Design review of the part shown in the three views and the two pictorial views. Dimensions are in mm from the part's minimum x, y and z. A direction names the side the tool comes from. Round coordinates to 2 decimals unless told otherwise and drop trailing zeros. Loops run counter-clockwise (first coordinate to the right, second up) from the corner with the lowest first, then second, coordinate; pieces in that order, holes last. Notation, with made-up numbers: (20.5, 74.5) -> (48.5, 74.5) arc R20 cw to (48.5, 81.5) -> close; hole circle Ø4 at (-35.5, -15). An arc over 180 degrees is marked (long way). Write each question's results on one line, items separated by ' | '. Start each with the question number.
Item 1: Clearance check with flat-ended pins moving along their axes: pin 1 Ø1.5 at (x, y) = (1.5, 18) entering from -Z; pin 2 Ø1.5 at (x, y) = (1, 18) entering from +Z; pin 3 Ø0.5 at (x, z) = (2, 0.5) entering from +Y. State where each tip first meets the part, or that it passes through.
Item 2: We need section A-A (z = 8). Give the boundary of the cut face in (x, y).
Item 3: Tool access review of the marked faces 1, 2, 3, 4 and 5: name each direction out of +Z, -Z, +X, -X, +Y, -Y from which nothing blocks a thin tool from reaching the whole face with its end or side.
Item 4: For L1, parallel to Y at x = 1.1, z = 8; L2, parallel to Z at x = 1.6, y = 16; L3, parallel to Y at x = 1.2, z = 9, list the stretches that pass through material, from the lowest coordinate up. Write a range as from..to.
Item 5: We need section B-B (x = 0.65). Give the boundary of the cut face in (y, z).
Item 6: We need section C-C (y = 28.5). Give the boundary of the cut face in (x, z).
Item 7: Mouldability with a two-part tool opening along Y and no side actions: class the marked faces 6, 7 and 8 as pulls with the +Y half, pulls with the -Y half, needs draft (parallel to the pull), parting line crosses it, or undercut.
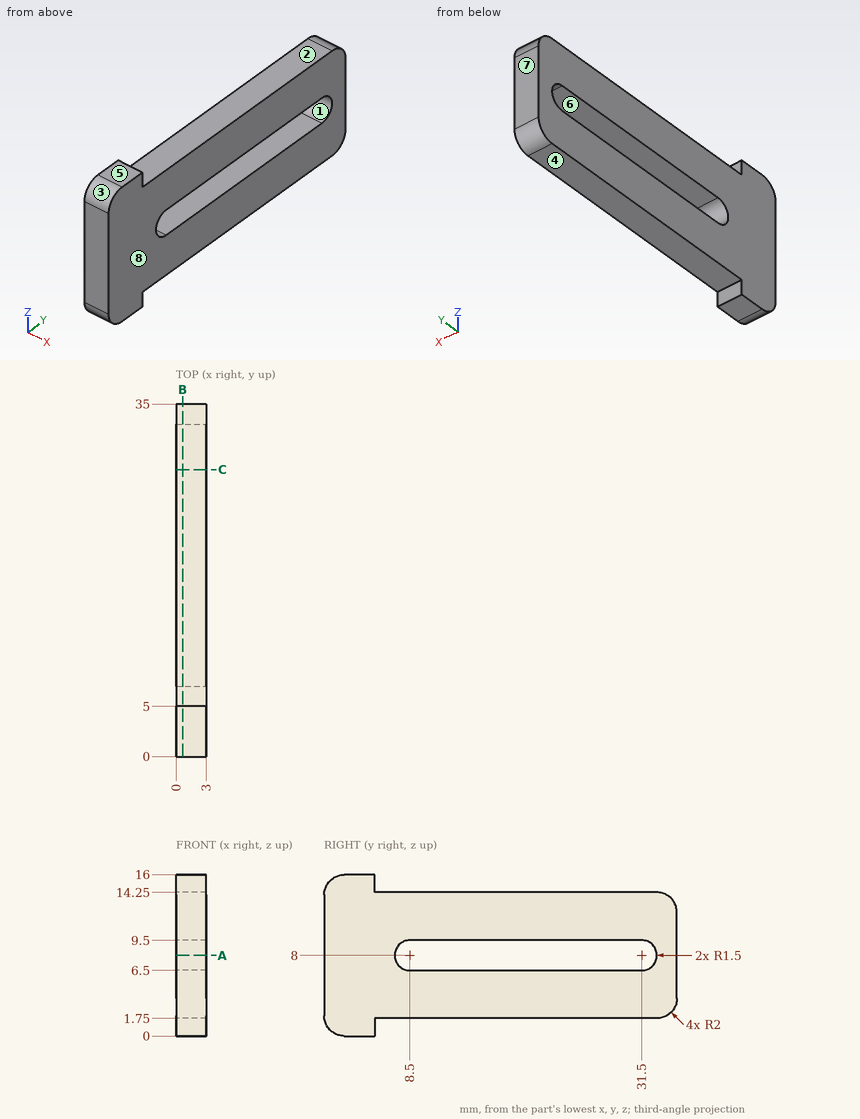
Here are the results:
1) pin 1: stops at z = 1.75 | pin 2: stops at z = 14.25 | pin 3: stops at y = 5
2) outline: (0, 0) -> (3, 0) -> (3, 7) -> (0, 7) -> close; (0, 33) -> (3, 33) -> (3, 35) -> (0, 35) -> close
3) face 1: +X, -X | face 2: +Z, +X, -X, +Y | face 3: +Z, +X, -X, -Y | face 4: -Z, +X, -X, +Y | face 5: +Z, +X, -X, +Y, -Y
4) L1: y = 0..7, 33..35 | L2: z = 1.75..6.5, 9.5..14.25 | L3: y = 0..7.38, 32.62..35
5) outline: (0, 2) arc R2 ccw to (2, 0) -> (5, 0) -> (5, 1.75) -> (33, 1.75) arc R2 ccw to (35, 3.75) -> (35, 12.25) arc R2 ccw to (33, 14.25) -> (5, 14.25) -> (5, 16) -> (2, 16) arc R2 ccw to (0, 14) -> close; hole (8.5, 6.5) -> (31.5, 6.5) arc R1.5 ccw to (31.5, 9.5) -> (8.5, 9.5) arc R1.5 ccw to start
6) outline: (0, 1.75) -> (3, 1.75) -> (3, 6.5) -> (0, 6.5) -> close; (0, 9.5) -> (3, 9.5) -> (3, 14.25) -> (0, 14.25) -> close
7) face 6: undercut | face 7: pulls with the +Y half | face 8: needs draft
